```python
from build123d import *

# Parameters (mm, degrees)
SKETCH1_W           = 108
SKETCH1_H           = 108
BOSS_EXTRUDE1_DEPTH = 170.1
SKETCH2_OUTSIDE_W   = 155.722
SKETCH2_OUTSIDE_H   = 155.722
SKETCH2_OUTSIDE_R   = 25.4
CUT_EXTRUDE1_DEPTH  = 6
SKETCH3_OUTSIDE_W   = 155.722
SKETCH3_OUTSIDE_H   = 155.722
SKETCH3_OUTSIDE_R   = 25.4
CUT_EXTRUDE3_DEPTH  = 163.1
SKETCH5_R           = 24.65
CUT_EXTRUDE4_DEPTH  = 187.456456043


with BuildPart() as part:
    # Sketch1 → Boss-Extrude1 (new body)
    with BuildSketch(Plane(origin=(0, 0, 0), x_dir=(1, 0, 0), z_dir=(0, 1, 0))):
        Rectangle(SKETCH1_W, SKETCH1_H)
    extrude(amount=BOSS_EXTRUDE1_DEPTH)

    # Sketch2 outside → Cut-Extrude1 (cut)
    with BuildSketch(Plane(origin=(0, 170.1, 0), x_dir=(1, 0, 0), z_dir=(0, 1, 0))):
        Rectangle(SKETCH2_OUTSIDE_W, SKETCH2_OUTSIDE_H)
        with Locations(Location((0, 0, 0), (0, 0, 270))):
            Circle(SKETCH2_OUTSIDE_R, mode=Mode.SUBTRACT)
    extrude(amount=-CUT_EXTRUDE1_DEPTH, mode=Mode.SUBTRACT)

    # Sketch3 outside → Cut-Extrude3 (cut)
    with BuildSketch(Plane.XZ):
        Rectangle(SKETCH3_OUTSIDE_W, SKETCH3_OUTSIDE_H)
        with Locations(Location((0, 0, 0), (0, 0, 90))):
            Circle(SKETCH3_OUTSIDE_R, mode=Mode.SUBTRACT)
    extrude(amount=-CUT_EXTRUDE3_DEPTH, mode=Mode.SUBTRACT)

    # Sketch5 → Cut-Extrude4 (cut, through all)
    with BuildSketch(Plane.XZ):
        with Locations(Location((0, 0, 0), (0, 0, 270))):
            Circle(SKETCH5_R)
    extrude(amount=-CUT_EXTRUDE4_DEPTH, mode=Mode.SUBTRACT)


solid = part.part
```
Check sheet for the modelled part. Datum: model origin and axes. Units: mm. A direction names the side the tool comes from. Round coordinates to 2 decimals unless told otherwise and drop trailing zeros. Order: outer loops, then holes, each group sorted by start corner. A loop starts at its lowest first (then second) coordinate and runs counter-clockwise, first axis right, second up. Notation, with made-up numbers: M 20,89 L 79,89 A24 ccw 79,101 Z; hole C 27.25,-34.75 d6. An arc over 180 degrees is marked long. Answer in a Markdown table with one row per item.
(1) Material ranges on line 1 along X through (y, z) = (101.5, 0); line 2 along Z through (x, y) = (3.5, 156); line 3 along Y through (x, z) = (-14.5, 26.5), recorded low to high. Write a range as from..to.
Findings:
| item | result |
|---|---|
| line 1 | x = -25.4..-24.65, 24.65..25.4 |
| line 2 | z = -25.16..-24.4, 24.4..25.16 |
| line 3 | y = 163.1..164.1 |
(2) Section check D-D on x = -46. Record the boundary of the cut face in (y, z).
Findings:
| item | result |
|---|---|
| outline | M 163.1,-54 L 164.1,-54 L 164.1,54 L 163.1,54 Z |
(3) Section check B-B on z = 0. Record the boundary of the cut face in (x, y), plus the area to 3 significant figures.
Findings:
| item | result |
|---|---|
| outline | M -54,163.1 L -25.4,163.1 L -25.4,0 L -24.65,0 L -24.65,170.1 L -25.4,170.1 L -25.4,164.1 L -54,164.1 Z; M 24.65,0 L 25.4,0 L 25.4,163.1 L 54,163.1 L 54,164.1 L 25.4,164.1 L 25.4,170.1 L 24.65,170.1 Z |
| area | 312 mm^2 |
(4) Set-up check for faces 4 (the flat face through (-25, 0, -2)), 5 (the flat face through (23, 164.1, -13)), 6 (the cylindrical face through (15.456, 80.408, -20.157)): record each of +Z, -Z, +X, -X, +Y, -Y from which the full face is reachable in a straight line by a thin tool's end or side.
Findings:
| item | result |
|---|---|
| face 4 | +Z, -Z, +X, -X, -Y |
| face 5 | +Y |
| face 6 | -Y |
(5) Section check C-C on y = 44.5. Record the boundary of the cut face in (x, z).
Findings:
| item | result |
|---|---|
| outline | C 0,0 d50.8; hole C 0,0 d49.3 |
(6) Gauge pin test, flat ends, axial feed: pin 1 (8 mm diameter, centred on x = 24, y = 53, fed in from -Z); pin 2 (1.5 mm diameter, centred on x = -3, z = -35, fed in from +Y); pin 3 (5 mm diameter, centred on x = -38.5, z = 34.5, fed in from -Y). Record the tip position at first contact, or that the pin passes through.
Findings:
| item | result |
|---|---|
| pin 1 | stops at z = -15.66 |
| pin 2 | stops at y = 164.1 |
| pin 3 | stops at y = 163.1 |
(7) Draft check along X on faces 1 (the cylindrical face through (24.44, 83.86, 3.21)), 2 (the flat face through (23, 163.1, 13)), 3 (the cylindrical face through (-15.456, 167.142, -20.157)). Enter one of: +X half, -X half, draft (parallel to the pull), parting line (faces both ways), or undercut.
Findings:
| item | result |
|---|---|
| face 1 | undercut |
| face 2 | draft |
| face 3 | parting line |
(8) Section check A-A on x = 0. Record the boundary of the cut face in (y, z), plus the area to 3 significant figures.
Findings:
| item | result |
|---|---|
| outline | M 0,-25.4 L 163.1,-25.4 L 163.1,-54 L 164.1,-54 L 164.1,-25.4 L 170.1,-25.4 L 170.1,-24.65 L 0,-24.65 Z; M 0,24.65 L 170.1,24.65 L 170.1,25.4 L 164.1,25.4 L 164.1,54 L 163.1,54 L 163.1,25.4 L 0,25.4 Z |
| area | 312 mm^2 |
